Can you work these out from the model? Positions are in its coordinate system, mm. A direction names the side the tool comes from. Give positions to 0.01 mm unless a question says otherwise; leave off trailing zeros. Write each loop counter-clockwise with the first axis right and the second up, starting at its lowest first coordinate (ties: lowest second). Pieces come first, ordered by that corner, then holes.
1. Suppose I cut it at B-B (z = -31.5). Please give me the cut outline in (x, y), and give its area (3 significant figures).
2. Thinking about a two-plate mould opening in Z: for faces 1 (the flat face through (4, 15, -47.5)), 2 (the flat face through (0, 0, -1)), 3 (the flat face through (0, 12, 46.5)), which applies, pulls with the +Z half, pulls with the -Z half, needs draft (parallel to the pull), parting line crosses it, or undercut?
3. Suppose I cut it at A-A (y = 15). Please give me the cut outline in (x, z).
4. Suppose I cut it at D-D (x = -4). Please give me the cut outline in (y, z), and give its area (3 significant figures).
5. If I drill on probe 1 along Z at (x, y) = (-0.75, 3.5); probe 2 along X at (y, z) = (0.2, 31.5); probe 3 along Y at (x, z) = (0, -46.8), over which ranges is the centre line in solid material (lowest first)?
6. Suppose I cut it at C-C (y = 4). Please give me the cut outline in (x, z), and give its area (3 significant figures).
7. I'm going to push flat-ended pins straight in: pin 1 (4 mm diameter, centred on x = -2, z = 34.5, fed in from +Y); pin 2 (3 mm diameter, centred on x = 0, y = 15, fed in from +Z). Where does each tip first touch, or does it pass through?
8. On a 3-axis mill with a long thin cutter (end or side, diameter ignored), from which of +Z, -Z, +X, -X, +Y, -Y can I reach the whole of each face in a straight line? I mean faces 4 (the flat face through (0, 1, -1)), 5 (the cylindrical face through (0.54, 17.44, 46.99)). Say none if no direction works.
```python
from build123d import *

# Parameters (mm, degrees)
CROQUIS2_W              = 30
CROQUIS2_H              = 95
SALIENTE_EXTRUIR1_DEPTH = 1
CROQUIS5_W              = 30
CROQUIS5_H              = 29
SALIENTE_EXTRUIR2_DEPTH = 1
CROQUIS6_W              = 30
CROQUIS6_H              = 29
SALIENTE_EXTRUIR3_DEPTH = 1
CROQUIS7_R              = 2.5
CORTAR_EXTRUIR1_DEPTH   = 1
CORTAR_EXTRUIR2_START   = -1
CROQUIS8_R              = 2.5
CORTAR_EXTRUIR2_DEPTH   = 1
REDONDEO1_R             = 10
CROQUIS9_R              = 2
CORTAR_EXTRUIR3_DEPTH   = 1


with BuildPart() as part:
    # Croquis2 → Saliente-Extruir1 (new body)
    with BuildSketch(Plane(origin=(0, 0, 0), x_dir=(1, 0, 0), z_dir=(0, 1, 0))):
        Rectangle(CROQUIS2_W, CROQUIS2_H)
    extrude(amount=SALIENTE_EXTRUIR1_DEPTH)

    # Croquis5 → Saliente-Extruir2 (add)
    with BuildSketch(Plane.XY.offset(47.5)):
        with Locations((0, 15.5)):
            Rectangle(CROQUIS5_W, CROQUIS5_H)
    extrude(amount=-SALIENTE_EXTRUIR2_DEPTH)

    # Croquis6 → Saliente-Extruir3 (add)
    with BuildSketch(Plane(origin=(0, 0, -47.5), x_dir=(-1, 0, 0), z_dir=(0, 0, -1))):
        with Locations((0, 15.5)):
            Rectangle(CROQUIS6_W, CROQUIS6_H)
    extrude(amount=-SALIENTE_EXTRUIR3_DEPTH)

    # Croquis7 → Cortar-Extruir1 (cut)
    with BuildSketch(Plane(origin=(0, 0, -47.5), x_dir=(-1, 0, 0), z_dir=(0, 0, -1))):
        with Locations((0, 15)):
            Circle(CROQUIS7_R)
    extrude(amount=-CORTAR_EXTRUIR1_DEPTH, mode=Mode.SUBTRACT)

    # Croquis8 → Cortar-Extruir2 (cut)
    with BuildSketch(Plane.XY.offset(47.5).offset(CORTAR_EXTRUIR2_START)):
        with Locations(Location((0, 15, 0), (0, 0, 180))):
            Circle(CROQUIS8_R)
    extrude(amount=CORTAR_EXTRUIR2_DEPTH, mode=Mode.SUBTRACT)

    # Redondeo1
    redondeo1_edges = [part.edges().sort_by_distance(p)[0] for p in [
        (-15, 30, 47),
        (-15, 30, -47),
    ]]
    fillet(redondeo1_edges, radius=REDONDEO1_R)

    # Croquis9 → Cortar-Extruir3 (cut)
    with BuildSketch(Plane(origin=(0, 1, 0), x_dir=(1, 0, 0), z_dir=(0, 1, 0))):
        with Locations(Location((0, 31.5, 0), (0, 0, 270))):
            Circle(CROQUIS9_R)
        with Locations(Location((0, -31.5, 0), (0, 0, 90))):
            Circle(CROQUIS9_R)
    extrude(amount=-CORTAR_EXTRUIR3_DEPTH, mode=Mode.SUBTRACT)


solid = part.part
```
Checks:
1. outline: (-15, 0) - (-2, 0) - (-2, 1) - (-15, 1) - close; (2, 0) - (15, 0) - (15, 1) - (2, 1) - close
1. area: 26.0 mm2
2. face 1: pulls with the -Z half
2. face 2: needs draft
2. face 3: undercut
3. outline: (-15, -47.5) - (-2.5, -47.5) - (-2.5, -46.5) - (-15, -46.5) - close; (-15, 46.5) - (-2.5, 46.5) - (-2.5, 47.5) - (-15, 47.5) - close; (2.5, -47.5) - (15, -47.5) - (15, -46.5) - (2.5, -46.5) - close; (2.5, 46.5) - (15, 46.5) - (15, 47.5) - (2.5, 47.5) - close
4. outline: (0, -47.5) - (30, -47.5) - (30, -46.5) - (1, -46.5) - (1, 46.5) - (30, 46.5) - (30, 47.5) - (0, 47.5) - close
4. area: 153 mm2
5. probe 1: z = -47.5 to -46.5, 46.5 to 47.5
5. probe 2: x = -15 to -2, 2 to 15
5. probe 3: y = 0 to 12.5, 17.5 to 30
6. outline: (-15, -47.5) - (15, -47.5) - (15, -46.5) - (-15, -46.5) - close; (-15, 46.5) - (15, 46.5) - (15, 47.5) - (-15, 47.5) - close
6. area: 60.0 mm2
7. pin 1: stops at y = 1
7. pin 2: passes through
8. face 4: +X, -X, +Y
8. face 5: +Z, -Z
